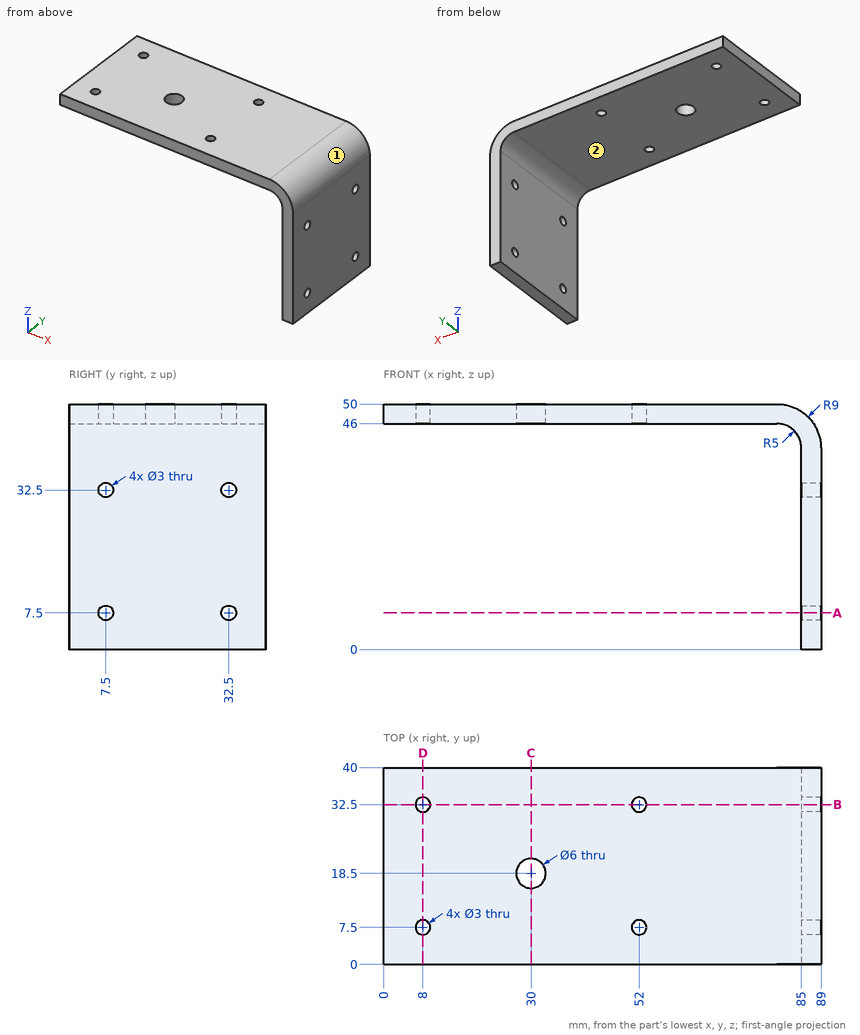
For this review, use the dimensioned drawing (mm, ordinates from the lowest corner) and the shaded views. A direction names the side the tool comes from. Give positions to 0.01 mm unless a question says otherwise; leave off trailing zeros. Order: outer loops, then holes, each group sorted by start corner. A loop starts at its lowest first (then second) coordinate and runs counter-clockwise, first axis right, second up. Notation, with made-up numbers: (-19, -12.75) - (-6, -12.75) arc R12 cw to (-6, -4.75) - close; hole circle Ø3 at (47.5, 76). An arc over 180 degrees is marked (long way). Use CSV: the item, a comma, the result in double quotes. Start each with the question number.
Q1. We need section D-D, the plane x = 8. Write out the cut boundary in (y, z), and give its area (3 significant figures).
Q2. Tool access review of the marked faces 1 and 2: name each direction out of +Z, -Z, +X, -X, +Y, -Y from which nothing blocks a thin tool from reaching the whole face with its end or side.
Q3. Clearance check with flat-ended pins moving along their axes: pin 1 Ø1 at (y, z) = (31.5, 32) entering from +X; pin 2 Ø1.8 at (x, y) = (8, 7.5) entering from +Z; pin 3 Ø9.5 at (x, y) = (30, 18.5) entering from -Z; pin 4 Ø3.5 at (y, z) = (32.5, 7.5) entering from -X. State where each tip first meets the part, or that it passes through.
Q4. We need section C-C, the plane x = 30. Write out the cut boundary in (y, z).
Q5. We need section B-B, the plane y = 32.5. Write out the cut boundary in (x, z), and give its area (3 significant figures).
Q6. To check wall thickness, follow line 1 along Y through (x, z) = (8, 49.15); line 2 along Z through (x, y) = (25.5, 4.5); line 3 along X through (y, z) = (22, 19.5). State the ranges of each line that lie inside material, in increasing order. Write a range as [from, to].
Q7. We need section A-A, the plane z = 7.5. Write out the cut boundary in (x, y), and give its area (3 significant figures).
Outcome:
1,outline,"(0, 46) - (6, 46) - (6, 50) - (0, 50) - close; (9, 46) - (31, 46) - (31, 50) - (9, 50) - close; (34, 46) - (40, 46) - (40, 50) - (34, 50) - close"
1,area,"136 mm^2"
2,face 1,"+Z, +X, +Y, -Y"
2,face 2,"-Z, -X, +Y, -Y"
3,pin 1,"stops at x = 89"
3,pin 2,"passes through"
3,pin 3,"stops at z = 46"
3,pin 4,"stops at x = 85"
4,outline,"(0, 46) - (15.5, 46) - (15.5, 50) - (0, 50) - close; (21.5, 46) - (40, 46) - (40, 50) - (21.5, 50) - close"
5,outline,"(0, 46) - (6.5, 46) - (6.5, 50) - (0, 50) - close; (9.5, 46) - (50.5, 46) - (50.5, 50) - (9.5, 50) - close; (53.5, 46) - (80, 46) arc R5 cw to (85, 41) - (85, 34) - (89, 34) - (89, 41) arc R9 ccw to (80, 50) - (53.5, 50) - close; (85, 0) - (89, 0) - (89, 6) - (85, 6) - close; (85, 9) - (89, 9) - (89, 31) - (85, 31) - close"
5,area,"480 mm^2"
6,line 1,"y = [0, 6], [9, 31], [34, 40]"
6,line 2,"z = [46, 50]"
6,line 3,"x = [85, 89]"
7,outline,"(85, 0) - (89, 0) - (89, 6) - (85, 6) - close; (85, 9) - (89, 9) - (89, 31) - (85, 31) - close; (85, 34) - (89, 34) - (89, 40) - (85, 40) - close"
7,area,"136 mm^2"
